from build123d import *
from build123d.topology import SkipClean

# Parameters (mm, degrees)
SKETCH1_R           = 35
BOSS_EXTRUDE1_DEPTH = 5
SKETCH2_R           = 1.6
CUT_EXTRUDE1_DEPTH  = 50.749371855
SKETCH3_R           = 6
BOSS_EXTRUDE2_DEPTH = 5
SKETCH6_R           = 4
CUT_EXTRUDE2_DEPTH  = 2


with BuildPart() as part:
    # Sketch1 → Boss-Extrude1 (new body)
    with BuildSketch(Plane(origin=(0, 0, 0), x_dir=(0, 0, -1), z_dir=(1, 0, 0))):
        Circle(SKETCH1_R)
        with BuildLine():
            Line((4, 6.92820323), (4, 24.677925359))
            ThreePointArc((4, 24.677925359), (17.67766953, 17.67766953), (24.677925359, 4))
            Line((24.677925359, 4), (6.92820323, 4))
            ThreePointArc((6.92820323, 4), (5.656854249, 5.656854249), (4, 6.92820323))
        make_face(mode=Mode.SUBTRACT)
        with BuildLine():
            Line((-4, 24.677925359), (-4, 6.92820323))
            ThreePointArc((-4, 6.92820323), (-5.656854249, 5.656854249), (-6.92820323, 4))
            Line((-6.92820323, 4), (-24.677925359, 4))
            ThreePointArc((-24.677925359, 4), (-17.67766953, 17.67766953), (-4, 24.677925359))
        make_face(mode=Mode.SUBTRACT)
        with BuildLine():
            Line((-24.677925359, -4), (-6.92820323, -4))
            ThreePointArc((-6.92820323, -4), (-5.656854249, -5.656854249), (-4, -6.92820323))
            Line((-4, -6.92820323), (-4, -24.677925359))
            ThreePointArc((-4, -24.677925359), (-17.67766953, -17.67766953), (-24.677925359, -4))
        make_face(mode=Mode.SUBTRACT)
        with BuildLine():
            Line((4, -24.677925359), (4, -6.92820323))
            ThreePointArc((4, -6.92820323), (5.656854249, -5.656854249), (6.92820323, -4))
            Line((6.92820323, -4), (24.677925359, -4))
            ThreePointArc((24.677925359, -4), (17.67766953, -17.67766953), (4, -24.677925359))
        make_face(mode=Mode.SUBTRACT)
        with BuildLine():
            Line((-2.28035085, 2.1), (2.28035085, 2.1))
            ThreePointArc((2.28035085, 2.1), (0, -3.1), (-2.28035085, 2.1))
        make_face(mode=Mode.SUBTRACT)
    extrude(amount=BOSS_EXTRUDE1_DEPTH)

    # Sketch2 → Cut-Extrude1 (cut, through all)
    with BuildSketch(Plane.ZY):
        with Locations((0, 30)):
            Circle(SKETCH2_R)
        with Locations((30, 0)):
            Circle(SKETCH2_R)
        with Locations((0, -30)):
            Circle(SKETCH2_R)
        with Locations((-30, 0)):
            Circle(SKETCH2_R)
    extrude(amount=-CUT_EXTRUDE1_DEPTH, mode=Mode.SUBTRACT)

    # Sketch3 → Boss-Extrude2 (add)
    with SkipClean():  # the faces are left unmerged after this step: merging them gives an invalid solid
        with BuildSketch(Plane.ZY):
            with Locations(Location((0, 0, 0), (0, 0, 180))):
                Circle(SKETCH3_R)
            with BuildLine():
                Line((-2.28035085, 2.1), (2.28035085, 2.1))
                ThreePointArc((2.28035085, 2.1), (0, -3.1), (-2.28035085, 2.1))
            make_face(mode=Mode.SUBTRACT)
        extrude(amount=BOSS_EXTRUDE2_DEPTH)

    # Sketch6 → Cut-Extrude2 (cut)
    with SkipClean():  # the faces are left unmerged after this step: merging them gives an invalid solid
        with BuildSketch(Plane.ZY):
            with Locations((0, 30)):
                Circle(SKETCH6_R)
            with Locations((30, 0)):
                Circle(SKETCH6_R)
            with Locations((0, -30)):
                Circle(SKETCH6_R)
            with Locations((-30, 0)):
                Circle(SKETCH6_R)
        extrude(amount=-CUT_EXTRUDE2_DEPTH, mode=Mode.SUBTRACT)


solid = part.part
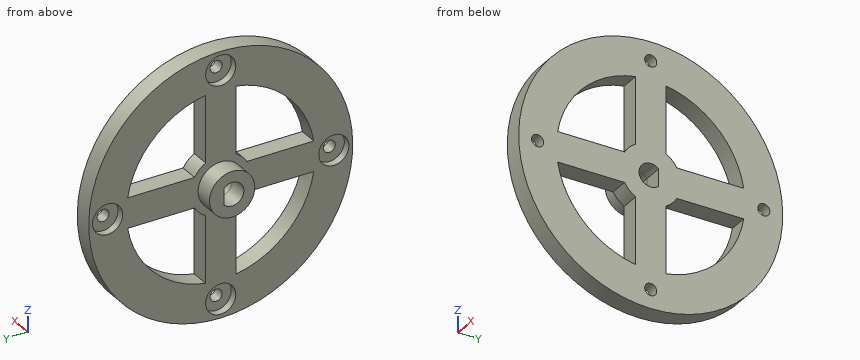
Geometry: final body of the model. Coordinates: model frame, mm. Give positions to 0.01 mm unless a question says otherwise; leave off trailing zeros. Loops run counter-clockwise (first coordinate to the right, second up) from the corner with the lowest first, then second, coordinate; pieces in that order, holes last. Notation, with made-up numbers: (45, -9.75) - (75, -9.75) arc R10 cw to (75, -2.75) - close; hole circle Ø4 at (87.25, 32). An arc over 180 degrees is marked (long way). One line per question, with ' | ' between items. Start each with the question number.
(1) Section query A-A on y = -30. Return loops of the section in (x, z).
(2) Ray query, line 1 (Y direction, x = 2.3, z = 0); line 2 (Y direction, x = 1.45, z = 0); line 3 (Y direction, x = -2.9, z = 0). Return the intervals inside material, ascending. Write a range as from..to.
(3) Contact query for flat-ended pins moving along their axis: pin 1 (8 mm diameter, centred on y = 18.5, z = 16.5, fed in from -X); pin 2 (5 mm diameter, centred on x = -3.5, z = 0, fed in from -Y); pin 3 (5 mm diameter, centred on x = 0, y = -8, fed in from -Z); pin 4 (3.5 mm diameter, centred on y = 0, z = 0, fed in from -X) (3 decimals). Output: stop coordinate, or through.
(4) Section query B-B on x = 4. Count the separate pieces of the cut face and the enclosed holes in it, then the cut area to 3 significant figures.
(5) Section query C-C on z = 14. Return loops of the section in (x, y).
The answers:
1) outline: (0, -18.03) - (5, -18.03) - (5, -1.6) - (2, -1.6) - (2, -4) - (0, -4) - close; (0, 4) - (2, 4) - (2, 1.6) - (5, 1.6) - (5, 18.03) - (0, 18.03) - close
2) line 1: -35..-31.6, -28.4..-3.1, 2.1..28.4, 31.6..35 | line 2: -35..-34, -26..-3.1, 2.1..26, 34..35 | line 3: -6..-3.1, 2.1..6
3) pin 1: x = 0 | pin 2: y = -6 | pin 3: z = -34.57 | pin 4: through
4) separate pieces: 1 | enclosed holes: 9 | area: 2,580 mm2
5) outline: (0, -32.08) - (5, -32.08) - (5, -20.71) - (0, -20.71) - close; (0, -4) - (5, -4) - (5, 4) - (0, 4) - close; (0, 20.71) - (5, 20.71) - (5, 32.08) - (0, 32.08) - close
